CAD build for the part. Positions are in the model's coordinates, mm. Coordinates: 2 decimals unless noted, no trailing zeros. Order: outer loops, then holes, each group sorted by start corner. A loop starts at its lowest first (then second) coordinate and runs counter-clockwise, first axis right, second up.
from build123d import *

# Parameters (mm, degrees)
F1_DEPTH = 25.4


with BuildPart() as f1:
    # F0 (on Right) → F1 (new body)
    with BuildSketch(Plane.YZ):
        with BuildLine():
            Line((0, 11.630322), (-66.565119, 11.630322))
            Line((-66.565119, 11.630322), (-66.565119, -22.185242))
            Line((-66.565119, -22.185242), (-56.224159, -22.185242))
            ThreePointArc((-56.224159, -22.185242), (-45.207921, -11.169004), (-34.191684, -22.185242))
            Line((-34.191684, -22.185242), (13.935136, -22.185242))
            ThreePointArc((13.935136, -22.185242), (25.537794, -10.582583), (37.140453, -22.185242))
            Line((37.140453, -22.185242), (70.476905, -22.185242))
            Line((70.476905, -22.185242), (0, 11.630322))
        make_face()
    extrude(amount=F1_DEPTH)


solid = f1.part
1) Two-plate mould, pull along Y, no slides. Class faces 1 (the flat face through (13, 54, -22.185)), 2 (the flat face through (12.5, 35.7, -5.5)), 3 (the cylindrical face through (12.522, 25.283, -10.585)): released by +Y, released by -Y, zero draft, split by the parting line, or undercut.
2) Slice it at A-A (z = -18). List the corners of the cut face in (x, y).
3) Slice it at B-B (x = 19.75). List the corners of the cut face in (y, z).
4) Slice it at C-C (y = -45). List the corners of the cut face in (x, z).
5) Drill centre lines: probe 1 along Y at (x, z) = (2, -15); probe 2 along Y at (x, z) = (19, -18); probe 3 along Z at (x, y) = (3.75, 6.5). Where is each one in solid material? Low to high.
6) Pin check, flat tips, straight feed: P1, Ø4, axis at x = 15.5, z = 1.5, coming from the +Y side; P2, Ø12, axis at x = 8, y = 19.5, coming from the +Z side. Stop position of each tip, or through.
7) Slice it at D-D (z = -7). List the corners of the cut face in (x, y), plus the area to 3 significant figures.
Worked out:
1. face 1: zero draft
1. face 2: released by +Y
1. face 3: undercut
2. outline: (0, -66.57) - (25.4, -66.57) - (25.4, -55.4) - (0, -55.4) - close; (0, -35.02) - (25.4, -35.02) - (25.4, 14.72) - (0, 14.72) - close; (0, 36.36) - (25.4, 36.36) - (25.4, 61.75) - (0, 61.75) - close
3. outline: (-66.57, -22.19) - (-56.22, -22.19) arc R11.02 cw to (-34.19, -22.19) - (13.94, -22.19) arc R11.6 cw to (37.14, -22.19) - (70.48, -22.19) - (0, 11.63) - (-66.57, 11.63) - close
4. outline: (0, -11.17) - (25.4, -11.17) - (25.4, 11.63) - (0, 11.63) - close
5. probe 1: y = -66.57 to -53.56, -36.86 to 16.43, 34.65 to 55.5
5. probe 2: y = -66.57 to -55.4, -35.02 to 14.72, 36.36 to 61.75
5. probe 3: z = -22.19 to 8.51
6. P1: stops at y = 25.28
6. P2: stops at z = 5.15
7. outline: (0, -66.57) - (25.4, -66.57) - (25.4, 38.83) - (0, 38.83) - close
7. area: 2,680 mm2
